Geometry check sheet. Reference: the model listing, model coordinates, mm. Give positions to 0.01 mm unless a question says otherwise; leave off trailing zeros. Loops run counter-clockwise (first coordinate to the right, second up) from the corner with the lowest first, then second, coordinate; pieces in that order, holes last. Notation, with made-up numbers: (-10.75, -25.75) - (-5.75, -25.75) arc R15 cw to (-5.75, -1.75) - close; hole circle Ø9 at (6.25, 60.5). An arc over 180 degrees is marked (long way). Use a Markdown table: item, result. Add a question column.
1. Cross-section at B-B on y = 29.5. Count the separate pieces of the cut face and the enclosed holes in it, and give its area (3 significant figures).
2. Cross-section at A-A on x = 7. Enter the section's corners in (y, z), and give its area (3 significant figures).
3. Depth check by flat-ended pin: P1, Ø8, axis at x = 22, y = 26, coming from the -Z side; P2, Ø1.5, axis at x = -2, z = -0.5, coming from the -Y side; P3, Ø4.5, axis at y = 1.5, z = 11, coming from the +X side; P4, Ø3, axis at y = 1.5, z = 15, coming from the -X side. Enter the tip coordinate at first touch or a pass-through.
4. Material ranges on L1, parallel to Y at x = 24, z = -5.5; L2, parallel to X at y = 3, z = 20.5; L3, parallel to Y at x = -5, z = -5, recorded low to high.
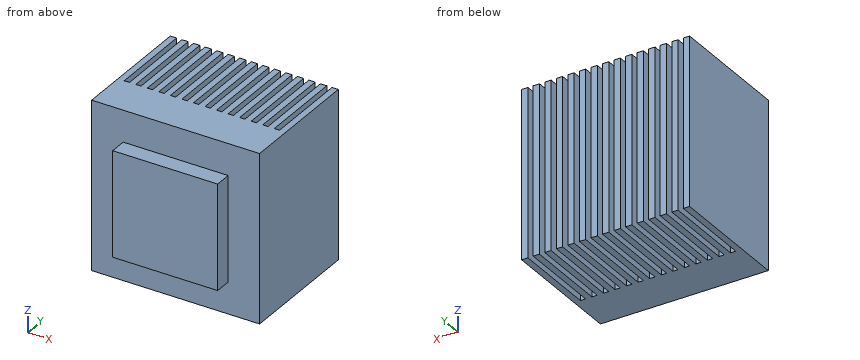
Autodesk Fusion 360 part; units mm, degrees
sketch "Sketch1" plane through (0, 0, 0) normal (0, 1, 0) x (1, 0, 0)
  line L0 (0, 0) -> (25, 0)
  line L1 (25, 0) -> (25, -25)
  line L2 (25, -25) -> (0, -25)
  line L3 (0, -25) -> (0, 0)
  dimension "d1" = 25
  dimension "d2" = 25
extrude "Extrude1" add sketch "Sketch1" along normal blind 4
sketch "Sketch2" plane through (0, 4, 0) normal (0, 1, 0) x (-1, 0, 0)
  line L0 (0, 25) -> (-25, 25)
  line L1 (-25, 25) -> (-25, 0)
  line L2 (-25, 0) -> (0, 0)
  line L3 (0, 0) -> (0, 25)
  line L4 (-32.5, 32.5) -> (-32.5, -7.5)
  line L5 (-32.5, -7.5) -> (7.5, -7.5)
  line L6 (7.5, -7.5) -> (7.5, 32.5)
  line L7 (7.5, 32.5) -> (-32.5, 32.5)
  line L8 (-32.5, 32.5) -> (-12.5, 32.5)
  dimension "d6" = 40
extrude "Extrude2" add sketch "Sketch2" along normal blind 10 contours L0 L1 L2 L3 | L4 L5 L6 L7 L8
sketch "Sketch3" plane through (0, 0, 32.5) normal (0, 0, 1) x (-1, 0, 0)
  line L0 (7.5, -4) -> (-32.5, -4)
  line L1 (-32.5, -4) -> (-32.5, -14)
  line L2 (-32.5, -14) -> (7.5, -14)
  line L3 (7.5, -14) -> (7.5, -4)
sketch "Sketch4" plane through (0, 0, 32.5) normal (0, 0, 1) x (-1, 0, 0)
  line L0 (7.5, -14) -> (7.5, -34)
  line L1 (7.5, -34) -> (5.5, -34)
  line L2 (5.5, -34) -> (5.5, -14)
  line L3 (5.5, -14) -> (7.5, -14)
  line L4 (3.28, -14) -> (3.28, -34)
  line L5 (3.28, -34) -> (1.28, -34)
  line L6 (1.28, -34) -> (1.28, -14)
  line L7 (-0.94, -14) -> (-0.94, -34)
  line L8 (-0.94, -34) -> (-2.94, -34)
  line L9 (-2.94, -34) -> (-2.94, -14)
  line L10 (-5.16, -14) -> (-5.16, -34)
  line L11 (-5.16, -34) -> (-7.16, -34)
  line L12 (-7.16, -34) -> (-7.16, -14)
  line L13 (-9.38, -14) -> (-9.38, -34)
  line L14 (-9.38, -34) -> (-11.38, -34)
  line L15 (-11.38, -34) -> (-11.38, -14)
  line L16 (-13.6, -14) -> (-13.6, -34)
  line L17 (-13.6, -34) -> (-15.6, -34)
  line L18 (-15.6, -34) -> (-15.6, -14)
  line L19 (-17.82, -14) -> (-17.82, -34)
  line L20 (-17.82, -34) -> (-19.82, -34)
  line L21 (-19.82, -34) -> (-19.82, -14)
  line L22 (-22.04, -14) -> (-22.04, -34)
  line L23 (-22.04, -34) -> (-24.04, -34)
  line L24 (-24.04, -34) -> (-24.04, -14)
  line L25 (-26.26, -14) -> (-26.26, -34)
  line L26 (-26.26, -34) -> (-28.26, -34)
  line L27 (-28.26, -34) -> (-28.26, -14)
  line L28 (-30.48, -14) -> (-30.48, -34)
  line L29 (-30.48, -34) -> (-32.48, -34)
  line L30 (-32.48, -34) -> (-32.48, -14)
  line L31 (7.5, -14) -> (-32.48, -14)
  line L32 (-32.48, -14) -> (7.5, -14)
  dimension "d11" = 20
  dimension "d12" = 2
  dimension "d15" = -4.22
  dimension "d16" = 0
sketch "Sketch5" plane through (0, 0, 32.5) normal (0, 0, 1) x (-1, 0, 0)
  line L0 (7.5, -14) -> (-32.5, -14)
  line L1 (7.5, -14) -> (7.5, -34)
  line L2 (7.5, -34) -> (6, -34)
  line L3 (6, -34) -> (6, -14)
  line L4 (7.5, -14) -> (6, -14)
  line L5 (4.75, -14) -> (4.75, -34)
  line L6 (3.25, -34) -> (3.25, -14)
  line L7 (4.75, -34) -> (3.25, -34)
  line L8 (2, -14) -> (2, -34)
  line L9 (0.5, -34) -> (0.5, -14)
  line L10 (2, -34) -> (0.5, -34)
  line L11 (-0.75, -14) -> (-0.75, -34)
  line L12 (-2.25, -34) -> (-2.25, -14)
  line L13 (-0.75, -34) -> (-2.25, -34)
  line L14 (-3.5, -14) -> (-3.5, -34)
  line L15 (-5, -34) -> (-5, -14)
  line L16 (-3.5, -34) -> (-5, -34)
  line L17 (-6.25, -14) -> (-6.25, -34)
  line L18 (-7.75, -34) -> (-7.75, -14)
  line L19 (-6.25, -34) -> (-7.75, -34)
  line L20 (-9, -14) -> (-9, -34)
  line L21 (-10.5, -34) -> (-10.5, -14)
  line L22 (-9, -34) -> (-10.5, -34)
  line L23 (-11.75, -14) -> (-11.75, -34)
  line L24 (-13.25, -34) -> (-13.25, -14)
  line L25 (-11.75, -34) -> (-13.25, -34)
  line L26 (-14.5, -14) -> (-14.5, -34)
  line L27 (-16, -34) -> (-16, -14)
  line L28 (-14.5, -34) -> (-16, -34)
  line L29 (-17.25, -14) -> (-17.25, -34)
  line L30 (-18.75, -34) -> (-18.75, -14)
  line L31 (-17.25, -34) -> (-18.75, -34)
  line L32 (-20, -14) -> (-20, -34)
  line L33 (-21.5, -34) -> (-21.5, -14)
  line L34 (-20, -34) -> (-21.5, -34)
  line L35 (-22.75, -14) -> (-22.75, -34)
  line L36 (-24.25, -34) -> (-24.25, -14)
  line L37 (-22.75, -34) -> (-24.25, -34)
  line L38 (-25.5, -14) -> (-25.5, -34)
  line L39 (-27, -34) -> (-27, -14)
  line L40 (-25.5, -34) -> (-27, -34)
  line L41 (-28.25, -14) -> (-28.25, -34)
  line L42 (-29.75, -34) -> (-29.75, -14)
  line L43 (-28.25, -34) -> (-29.75, -34)
  line L44 (-31, -14) -> (-31, -34)
  line L45 (-32.5, -34) -> (-32.5, -14)
  line L46 (-31, -34) -> (-32.5, -34)
  dimension "d19" = 20
  dimension "d22" = -2.75
  dimension "d23" = 0
extrude "Extrude4" add sketch "Sketch5" against normal blind 40
Values found:
| question | item | result |
|---|---|---|
| 1 | separate pieces | 15 |
| 1 | enclosed holes | 0 |
| 1 | area | 900 mm2 |
| 2 | outline | (0, 0) - (4, 0) - (4, -7.5) - (34, -7.5) - (34, 32.5) - (4, 32.5) - (4, 25) - (0, 25) - close |
| 2 | area | 1,300 mm2 |
| 3 | P1 | stops at z = -7.5 |
| 3 | P2 | stops at y = 4 |
| 3 | P3 | stops at x = 25 |
| 3 | P4 | stops at x = 0 |
| 4 | L1 | y = 4 to 34 |
| 4 | L2 | x = 0 to 25 |
| 4 | L3 | y = 4 to 14 |
